Can you work these out from the model? Positions are in its coordinate system, mm. A direction names the side the tool comes from. Coordinates: 2 decimals unless noted, no trailing zeros. Order: outer loops, then holes, each group sorted by start corner. A loop starts at its lowest first (then second) coordinate and runs counter-clockwise, first axis right, second up. Notation, with made-up numbers: (7.5, -18.5) -> (39.5, -18.5) arc R22 ccw to (39.5, -11.5) -> close; hole circle Ø11 at (60, 5). An arc over 180 degrees is marked (long way). Write item = value, one per line.
```python
from build123d import *

# Parameters (mm, degrees)
SKETCH1_R           = 2
BOSS_EXTRUDE1_DEPTH = 1.6
SKETCH1_3_W         = 8.2
SKETCH1_3_H         = 8.2
SKETCH1_3_W_2       = 6.2
SKETCH1_3_H_2       = 6.2
BOSS_EXTRUDE2_DEPTH = 2
BOSS_EXTRUDE3_START = -0.5
SKETCH1_4_W         = 8.2
SKETCH1_4_H         = 8.2
SKETCH1_4_W_2       = 6.2
SKETCH1_4_H_2       = 6.2
SKETCH1_4_R         = 2
BOSS_EXTRUDE3_DEPTH = 0.5
SKETCH3_W           = 5.8
SKETCH3_H           = 5.8
BOSS_EXTRUDE4_DEPTH = 4.5
CHAMFER1_SIZE       = 0.5
CUT_EXTRUDE1_DEPTH  = 0.2


with BuildPart() as part:
    # Sketch1 → Boss-Extrude1 (new body)
    with BuildSketch(Plane(origin=(0, 0, 0), x_dir=(1, 0, 0), z_dir=(0, 1, 0))):
        with Locations(Location((0, 0, 0), (0, 0, 270))):
            Circle(SKETCH1_R)
    extrude(amount=BOSS_EXTRUDE1_DEPTH)



with BuildPart() as body_2:
    # Sketch1_3 → Boss-Extrude2 (new body)
    with BuildSketch(Plane(origin=(0, 0, 0), x_dir=(1, 0, 0), z_dir=(0, 1, 0))):
        Rectangle(SKETCH1_3_W, SKETCH1_3_H)
        Rectangle(SKETCH1_3_W_2, SKETCH1_3_H_2, mode=Mode.SUBTRACT)
    extrude(amount=BOSS_EXTRUDE2_DEPTH)


with BuildPart() as part_1:
    add(part.part)

    add(body_2.part)  # Boss-Extrude3 merges body 2
    # Sketch1_4 → Boss-Extrude3 (add)
    # profile 1 of 3: a face of its own
    with BuildSketch(Plane(origin=(0, 0, 0), x_dir=(1, 0, 0), z_dir=(0, 1, 0)).offset(BOSS_EXTRUDE3_START)):
        Rectangle(SKETCH1_4_W, SKETCH1_4_H)
        Rectangle(SKETCH1_4_W_2, SKETCH1_4_H_2, mode=Mode.SUBTRACT)
    # profile 2 of 3: a face of its own
    with BuildSketch(Plane(origin=(0, 0, 0), x_dir=(1, 0, 0), z_dir=(0, 1, 0)).offset(BOSS_EXTRUDE3_START)):
        Rectangle(SKETCH1_4_W_2, SKETCH1_4_H_2)
        with Locations(Location((0, 0, 0), (0, 0, 270))):
            Circle(SKETCH1_4_R, mode=Mode.SUBTRACT)
    # profile 3 of 3: a face of its own
    with BuildSketch(Plane(origin=(0, 0, 0), x_dir=(1, 0, 0), z_dir=(0, 1, 0)).offset(BOSS_EXTRUDE3_START)):
        with Locations(Location((0, 0, 0), (0, 0, 270))):
            Circle(SKETCH1_4_R)
    extrude(amount=BOSS_EXTRUDE3_DEPTH)

    # Sketch3 → Boss-Extrude4 (add)
    with BuildSketch(Plane.XZ.offset(0.5)):
        Rectangle(SKETCH3_W, SKETCH3_H)
    extrude(amount=BOSS_EXTRUDE4_DEPTH)

    # Chamfer1
    chamfer1_edges = [part_1.edges().sort_by_distance(p)[0] for p in [
        (2.9, -2.75, -2.9),
        (2.9, -2.75, 2.9),
        (-2.9, -2.75, 2.9),
        (-2.9, -2.75, -2.9),
        (-4.1, 0.75, -4.1),
        (4.1, 0.75, -4.1),
        (4.1, 0.75, 4.1),
        (-4.1, 0.75, 4.1),
    ]]
    chamfer(chamfer1_edges, length=CHAMFER1_SIZE)

    # Sketch4 → Cut-Extrude1 (cut)
    with BuildSketch(Plane.XZ.offset(5)):
        with BuildLine():
            Line((-0.866374082, 1.850562538), (-0.165953409, 1.850562538))
            add(Edge.make_bspline(
                [(-0.165953409, 1.850562538), (-0.11921228, 1.850406952), (-0.029464136, 1.85010821), (0.099109135, 1.848442447), (0.215936232, 1.843668091), (0.320956071, 1.839559508), (0.414166726, 1.832067567), (0.495854017, 1.824906919), (0.565641714, 1.815533259), (0.607887566, 1.806827836), (0.627015341, 1.802886256)],
                knots=[0, 0, 0, 0, 1.410062039, 2.707475311, 3.878576406, 4.937260626, 5.877586885, 6.699081471, 7.410979367, 8, 8, 8, 8], degree=3))
            add(Edge.make_bspline(
                [(0.627015341, 1.802886256), (0.652621966, 1.796559491), (0.703288955, 1.784040927), (0.776239021, 1.757581326), (0.845753345, 1.726961702), (0.911543169, 1.690997981), (0.973278961, 1.649423202), (1.031597271, 1.602955079), (1.086762735, 1.551847874), (1.136544365, 1.494813032), (1.183483417, 1.434976522), (1.223072043, 1.370272766), (1.257198523, 1.302611238), (1.28436904, 1.23130382), (1.306247013, 1.157042048), (1.321673253, 1.079153252), (1.33092444, 0.997992277), (1.331866296, 0.942634368), (1.332343867, 0.914564942)],
                knots=[0, 0, 0, 0, 1.027469482, 2.033020251, 3.019912614, 3.986113645, 4.951240523, 5.91722682, 6.890402269, 7.87763091, 8.8651537, 9.85103654, 10.82876324, 11.815024772, 12.821070561, 13.842952187, 14.906261191, 16, 16, 16, 16], degree=3))
            add(Edge.make_bspline(
                [(1.332343867, 0.914564942), (1.330874869, 0.867929837), (1.328008473, 0.77693267), (1.30128337, 0.644871788), (1.25750685, 0.521682474), (1.197183561, 0.407519836), (1.120364085, 0.30460919), (1.028039294, 0.214218735), (0.920157682, 0.138578822), (0.819728367, 0.086126018), (0.731014167, 0.052533109), (0.657980854, 0.02889675), (0.578313877, 0.010634785), (0.492776542, -0.005725347), (0.401012886, -0.018077041), (0.303242847, -0.027123636), (0.199396695, -0.032777684), (0.128057626, -0.033619689), (0.09135829, -0.034052846)],
                knots=[0, 0, 0, 0, 1.260483769, 2.459530307, 3.627416485, 4.787058657, 5.939039949, 7.08810263, 8.267026773, 9.491475466, 10.141966685, 10.831826277, 11.566392101, 12.351337768, 13.187381173, 14.07005841, 15.007169909, 16, 16, 16, 16], degree=3))
            Line((0.09135829, -0.034052846), (1.377215662, -1.649437462))
            Line((1.377215662, -1.649437462), (0.988794188, -1.649437462))
            Line((0.988794188, -1.649437462), (-0.297063184, -0.034052846))
            Line((-0.297063184, -0.034052846), (-0.552271517, -0.034052846))
            Line((-0.552271517, -0.034052846), (-0.552271517, -1.649437462))
            Line((-0.552271517, -1.649437462), (-0.866374082, -1.649437462))
            Line((-0.866374082, -1.649437462), (-0.866374082, 1.850562538))
        make_face()
        with BuildLine():
            Line((-0.552271517, 1.491588179), (-0.552271517, 0.324921513))
            Line((-0.552271517, 0.324921513), (0.088553803, 0.32001366))
            add(Edge.make_bspline(
                [(0.088553803, 0.32001366), (0.118473842, 0.320000423), (0.176467399, 0.319974767), (0.260368064, 0.323968543), (0.338488176, 0.328511861), (0.410528928, 0.335461207), (0.476522503, 0.344417279), (0.536435916, 0.355620263), (0.590366968, 0.368672326), (0.653265507, 0.388873951), (0.723502038, 0.42087997), (0.799833498, 0.467445468), (0.864835836, 0.526014588), (0.919753698, 0.592988044), (0.963883129, 0.666624292), (0.994995184, 0.746040662), (1.014737626, 0.82923226), (1.017066171, 0.886410367), (1.018241303, 0.915266064)],
                knots=[0, 0, 0, 0, 1.146690395, 2.22261258, 3.21895312, 4.145990853, 4.996080663, 5.770904154, 6.481378293, 7.121626537, 8.300444488, 9.431385265, 10.535395872, 11.636531494, 12.74115979, 13.810798291, 14.895190096, 16, 16, 16, 16], degree=3))
            add(Edge.make_bspline(
                [(1.018241303, 0.915266064), (1.017039182, 0.943412638), (1.014657017, 0.999188876), (0.995208248, 1.080844787), (0.962318867, 1.157911737), (0.917996629, 1.230076222), (0.863997474, 1.295581958), (0.800679661, 1.351629111), (0.729774466, 1.397878575), (0.663503268, 1.427432956), (0.604269055, 1.445552809), (0.552839395, 1.458303973), (0.494727917, 1.468548442), (0.429652459, 1.476756503), (0.357890828, 1.483811447), (0.279080177, 1.488563226), (0.193743397, 1.49137709), (0.134596465, 1.491516179), (0.103978483, 1.491588179)],
                knots=[0, 0, 0, 0, 1.101028733, 2.181837193, 3.264309656, 4.369019818, 5.486613113, 6.575447106, 7.666700264, 8.788928104, 9.402425223, 10.0903467, 10.862060571, 11.710948788, 12.657782767, 13.684531032, 14.801375019, 16, 16, 16, 16], degree=3))
            Line((0.103978483, 1.491588179), (-0.552271517, 1.491588179))
        make_face(mode=Mode.SUBTRACT)
    extrude(amount=-CUT_EXTRUDE1_DEPTH, mode=Mode.SUBTRACT)


solid = part_1.part
```
Item 1: I want a section at D-D, the plane x = -1.5. Please give me the cut outline in (y, z).
A:
outline = (-5, -2.9) -> (-0.5, -2.9) -> (-0.5, -4.1) -> (2, -4.1) -> (2, -3.1) -> (0, -3.1) -> (0, -1.32) -> (1.6, -1.32) -> (1.6, 1.32) -> (0, 1.32) -> (0, 3.1) -> (2, 3.1) -> (2, 4.1) -> (-0.5, 4.1) -> (-0.5, 2.9) -> (-5, 2.9) -> close
Item 2: I want a section at A-A, the plane y = 1.75. Please give me the cut outline in (x, z), plus the area to 3 significant figures.
A:
outline = (-4.1, -3.6) -> (-3.6, -4.1) -> (3.6, -4.1) -> (4.1, -3.6) -> (4.1, 3.6) -> (3.6, 4.1) -> (-3.6, 4.1) -> (-4.1, 3.6) -> close; hole (-3.1, -3.1) -> (3.1, -3.1) -> (3.1, 3.1) -> (-3.1, 3.1) -> close
area = 28.3 mm2
Item 3: If we mould it in two halves opening along Z, with no side actions, what happens to faces 5 (the cylindrical face through (-2, 1, 0)), 6 (the flat face through (-4.1, 1, 0)), 7 (the flat face through (0, 1, 3.1)), 8 (the flat face through (0, 1, 4.1))? For each: pulls with the +Z half, pulls with the -Z half, needs draft (parallel to the pull), parting line crosses it, or undercut.
A:
face_5 = undercut
face_6 = needs draft
face_7 = undercut
face_8 = pulls with the +Z half
Item 4: I'm going to push flat-ended pins straight in: P1, Ø3, axis at x = -3, y = -2.5, coming from the -Z side; P2, Ø1.5, axis at y = -2.5, z = -2.5, coming from the -X side; P3, Ø1.2, axis at x = 0.5, z = 0.5, coming from the +Y side. Where does each tip first touch, or does it pass through?
A:
P1 = -2.9
P2 = -2.9
P3 = 1.6
Item 5: I want a section at C-C, the plane z = 3.25. Please give me the cut outline in (x, y), plus the area to 3 significant figures.
A:
outline = (-4.1, -0.5) -> (4.1, -0.5) -> (4.1, 2) -> (-4.1, 2) -> close
area = 20.5 mm2
Item 6: I want a section at B-B, the plane y = -3. Please give me the cut outline in (x, z).
A:
outline = (-2.9, -2.4) -> (-2.4, -2.9) -> (2.4, -2.9) -> (2.9, -2.4) -> (2.9, 2.4) -> (2.4, 2.9) -> (-2.4, 2.9) -> (-2.9, 2.4) -> close
Item 7: If I drill on probe 1 along Z at (x, y) = (1.75, 1.25); probe 2 along Z at (x, y) = (2.75, 0.75), over which ranges is the centre line in solid material (lowest first)?
A:
probe_1 = -4.1 to -3.1, -0.97 to 0.97, 3.1 to 4.1
probe_2 = -4.1 to -3.1, 3.1 to 4.1
Item 8: For faces 1 (the flat face through (0, -3, 2.9)), 2 (the flat face through (0, -3, -2.9)), 3 (the flat face through (-3.1, 1, 0)), 4 (the flat face through (-3.7, -0.5, -0.1)), which set-ups out of +Z, -Z, +X, -X, +Y, -Y let a thin tool reach every point of the face, with its end or its side?
A:
face_1 = +Z, +X, -X, -Y
face_2 = -Z, +X, -X, -Y
face_3 = +Y
face_4 = -Y
